Model file for the job. Use its own axes, mm. A direction names the side the tool comes from. Coordinates: 2 decimals unless noted, no trailing zeros. Loops run counter-clockwise (first coordinate to the right, second up) from the corner with the lowest first, then second, coordinate; pieces in that order, holes last. Notation, with made-up numbers: M -36,85 L 21,85 A25 ccw 21,109 Z; hole C 46.5,46 d8. An arc over 180 degrees is marked long. Write item = value, one per line. Start each with the question number.
Autodesk Inventor part; units mm, degrees
ref_plane "YZ Plane" through (0, 0, 0) normal (1, 0, 0) x (0, 1, 0)
ref_plane "XZ Plane" through (0, 0, 0) normal (0, 1, 0) x (-1, 0, 0)
ref_plane "XY Plane" through (0, 0, 0) normal (0, 0, 1) x (1, 0, 0)
sketch "Sketch1" plane through (0, 0, 0) normal (0, 0, 1) x (1, 0, 0)
  line L0 (-15.35, 11.85) -> (15.35, 11.85)
  line L1 (15.35, 11.85) -> (15.35, -11.85)
  line L2 (15.35, -11.85) -> (-15.35, -11.85)
  line L3 (-15.35, -11.85) -> (-15.35, 11.85)
  point P0 (0, 0)
  dimension "d0" = 30.7
  dimension "d2" = 23.7
  dimension "d3" = 15.35
  dimension "d4" = 11.85
extrude "Extrusion1" add sketch "Sketch1" against normal blind 3.2
sketch "Sketch2" plane through (0, 0, -3.2) normal (0, 0, -1) x (-1, 0, 0)
  line L0 (15.35, -11.85) -> (15.35, 11.85)
  line L1 (-11.25, 9.9) -> (11.25, 9.9)
  line L2 (13.25, 6.2453) -> (13.25, -5.9)
  line L3 (11.75, -9.9) -> (-11.75, -9.9)
  line L4 (-13.25, -5.9) -> (-13.25, 6.2453)
  line L5 (11.75, -9.9) -> (11.75, -9.0225)
  arc A0 (11.75, -9.0225) -> (13.25, -5.9) centre (9.25, -5.9) ccw
  line L6 (0, 0) -> (0, 2.1839)
  line L7 (-11.75, -9.9) -> (-11.75, -9.0225)
  arc A1 (-13.25, -5.9) -> (-11.75, -9.0225) centre (-9.25, -5.9) ccw
  line L8 (11.25, 9.9) -> (11.25, 7.4)
  line L9 (11.25, 7.4) -> (13.25, 6.2453)
  line L10 (-11.25, 9.9) -> (-11.25, 7.4)
  line L11 (-11.25, 7.4) -> (-13.25, 6.2453)
  dimension "d10" = 9.9
  dimension "d11" = 13.25
  dimension "d13" = 8
  dimension "d15" = 1.5
  dimension "d19" = 120
  dimension "d20" = 19.8
  dimension "d21" = 2
  dimension "d22" = 2.5
extrude "Extrusion2" add sketch "Sketch2" along normal blind 16
sketch "Sketch3" plane through (0, 0, -19.2) normal (0, 0, -1) x (-1, 0, 0)
  line L0 (-11.25, 9.9) -> (-11.25, 7.4)
  line L1 (-1.75, 7.5) -> (-1.75, -0.5)
  line L2 (-1.75, -0.5) -> (1.75, -0.5)
  line L3 (1.75, -0.5) -> (1.75, 7.5)
  line L4 (1.75, 7.5) -> (-1.75, 7.5)
  line L5 (-9.5, 2) -> (-9.5, -6)
  line L6 (-9.5, -6) -> (-6, -6)
  line L7 (-6, -6) -> (-6, 2)
  line L8 (-6, 2) -> (-9.5, 2)
  line L9 (6, 2) -> (6, -6)
  line L10 (6, -6) -> (9.5, -6)
  line L11 (9.5, -6) -> (9.5, 2)
  line L12 (9.5, 2) -> (6, 2)
  point P0 (0, 0)
  dimension "d25" = 3.5
  dimension "d27" = 8
  dimension "d28" = 1.75
  dimension "d29" = 7.5
  dimension "d30" = 3.5
  dimension "d31" = 8
  dimension "d32" = 3.5
  dimension "d33" = 8
  dimension "d34" = 2
  dimension "d35" = 2
  dimension "d36" = 6
  dimension "d37" = 6
extrude "Extrusion3" add sketch "Sketch3" along normal blind 1.5
sketch "Sketch4" plane through (0, 0, -20.7) normal (0, 0, -1) x (-1, 0, 0)
  line L0 (-6, -6) -> (-6, 2)
  line L1 (-6, 2) -> (-9.5, 2)
  line L2 (-8.25, 0) -> (-8.25, -4)
  line L3 (-8.25, -4) -> (-7.25, -4)
  line L4 (-7.25, -4) -> (-7.25, 0)
  line L5 (-7.25, 0) -> (-8.25, 0)
  point P0 (-9.5, -6)
  point P1 (0, 0)
  dimension "d40" = 4
  dimension "d42" = 1
  dimension "d43" = 1.25
  dimension "d44" = 3.5
  dimension "d45" = 8
  dimension "d46" = 2
extrude "Extrusion4" add sketch "Sketch4" along normal blind 5.5
sketch "Sketch6" plane through (0, 0, -20.7) normal (0, 0, -1) x (-1, 0, 0)
  line L0 (-1.75, -0.5) -> (1.75, -0.5)
  line L1 (1.75, -0.5) -> (1.75, 7.5)
  line L2 (1.75, 7.5) -> (-1.75, 7.5)
  line L3 (-0.5, 5.5) -> (0.5, 5.5)
  line L4 (0.5, 5.5) -> (0.5, 1.5)
  line L5 (0.5, 1.5) -> (-0.5, 1.5)
  line L6 (-0.5, 1.5) -> (-0.5, 5.5)
  point P0 (0, 0)
  dimension "d55" = 1
  dimension "d57" = 4
  dimension "d58" = 1.25
  dimension "d59" = 2
  dimension "d60" = 8
  dimension "d61" = 2
extrude "Extrusion5" add sketch "Sketch6" along normal blind 5.5
sketch "Sketch7" plane through (0, 0, -20.7) normal (0, 0, -1) x (-1, 0, 0)
  line L0 (9.5, -6) -> (9.5, 2)
  line L1 (9.5, 2) -> (6, 2)
  line L2 (8.25, -4) -> (7.25, -4)
  line L3 (7.25, -4) -> (7.25, 0)
  line L4 (7.25, 0) -> (8.25, 0)
  line L5 (8.25, 0) -> (8.25, -4)
  point P0 (0, 0)
  dimension "d64" = 2
  dimension "d65" = 4
  dimension "d66" = 1.25
  dimension "d67" = 1
extrude "Extrusion6" add sketch "Sketch7" along normal blind 5.5
sketch "Sketch8" plane through (8.25, -4, -20.7) normal (1, 0, 0) x (0, 0, -1)
  line L0 (0, 0) -> (0, 4)
  line L1 (0, 0) -> (5.5, 0)
  line L2 (5.5, 4) -> (5.5, 0)
  line L3 (0, 4) -> (5.5, 4)
  arc A0 (3.5, 0) -> (3.5, 4) centre (3.5, 2) ccw
  arc A1 (3.5, 0.9) -> (3.5, 3.1) centre (3.5, 2) ccw
  line L4 (3.5, 2) -> (2.8, 2)
  arc A2 (2.8, 3.1) -> (2.8, 0.9) centre (2.8, 2) ccw
  line L5 (2.8, 3.1) -> (3.5, 3.1)
  line L6 (3.5, 0.9) -> (2.8, 0.9)
  line L7 (3.5, 4) -> (5.5, 4)
  line L8 (5.5, 4) -> (5.5, 0)
  line L9 (5.5, 0) -> (3.5, 0)
  point P0 (-20.7, 4)
  dimension "d70" = 4
  dimension "d72" = 2.2
  dimension "d73" = 0.7
  dimension "d74" = 2.2
extrude "Extrusion7" cut sketch "Sketch8" against normal blind 1 contours A0 L2 L1 | L3 L2 A0 | L6 A2 L5 A1
sketch "Sketch11" plane through (0.5, 1.5, -20.7) normal (1, 0, 0) x (0, 0, -1)
  line L0 (0, 0) -> (0, 4)
  line L1 (0, 0) -> (5.5, 0)
  line L2 (5.5, 4) -> (5.5, 0)
  line L3 (0, 4) -> (5.5, 4)
  arc A0 (3.5, 0) -> (3.5, 4) centre (3.5, 2) ccw
  line L4 (3.5, 0) -> (5.5, 0)
  line L5 (5.5, 4) -> (5.5, 0)
  line L6 (5.5, 4) -> (3.5, 4)
  arc A1 (3.5, 0.9) -> (3.5, 3.1) centre (3.5, 2) ccw
  line L7 (3.5, 2) -> (2.8, 2)
  arc A2 (2.8, 3.1) -> (2.8, 0.9) centre (2.8, 2) ccw
  line L8 (2.8, 3.1) -> (3.5, 3.1)
  line L9 (3.5, 0.9) -> (2.8, 0.9)
  point P0 (-20.7, -1.5)
  dimension "d88" = 4
  dimension "d91" = 2.2
  dimension "d92" = 0.7
  dimension "d93" = 2.2
sketch "Sketch12" plane through (-7.25, -4, -20.7) normal (1, 0, 0) x (0, 0, -1)
  arc A0 (3.5, 0) -> (3.5, 4) centre (3.5, 2) ccw
  arc A1 (3.5, 0.9) -> (3.5, 3.1) centre (3.5, 2) ccw
  line L0 (3.5, 2) -> (2.8, 2)
  arc A2 (2.8, 3.1) -> (2.8, 0.9) centre (2.8, 2) ccw
  line L1 (2.8, 3.1) -> (3.5, 3.1)
  line L2 (3.5, 0.9) -> (2.8, 0.9)
  line L3 (0, 4) -> (5.5, 4)
  line L4 (5.5, 4) -> (5.5, 0)
  line L5 (5.5, 4) -> (3.5, 4)
  line L6 (3.5, 0) -> (5.5, 0)
  point P0 (-20.7, -1.5)
  dimension "d94" = 4
  dimension "d95" = 2.2
  dimension "d96" = 0.7
  dimension "d97" = 2.2
extrude "Extrusion8" cut sketch "Sketch11" against normal blind 1 contours A0 L2 L1 | L3 L2 A0 | L9 A2 L8 A1
extrude "Extrusion9" cut sketch "Sketch12" against normal blind 1 contours L2 A2 L1 A1
sketch "Sketch13" plane through (-7.25, -4, -20.7) normal (1, 0, 0) x (0, 0, -1)
  line L0 (0, 0) -> (5.5, 0)
  line L1 (5.5, 4) -> (5.5, 0)
  line L2 (0, 4) -> (5.5, 4)
  circle A0 centre (3.5, 2) radius 2
  line L3 (3.5, 4) -> (5.5, 4)
  line L4 (5.5, 0) -> (5.5, 4)
  line L5 (3.5, 0) -> (5.5, 0)
  point P0 (-20.7, 4)
  dimension "d102" = 4
extrude "Extrusion10" cut sketch "Sketch13" against normal blind 1 contours A0 L1 L0 | L2 L1 A0
sketch "Sketch14" plane through (0, 0, 0) normal (0, 0, 1) x (1, 0, 0)
  line L0 (12, -8) -> (-12, -8)
  line L1 (-7, 8) -> (7, 8)
  line L2 (12, 3) -> (12, -8)
  line L3 (7, 8) -> (12, 3)
  line L4 (0, 0) -> (0, 4.7583)
  line L5 (-7, 8) -> (-12, 3)
  line L6 (-12, -8) -> (-12, 3)
  dimension "d107" = 16
  dimension "d108" = 12
  dimension "d109" = 8
  dimension "d110" = 45
  dimension "d111" = 5
extrude "Extrusion11" cut sketch "Sketch14" against normal blind 16
fillet "Fillet1" radius 1.5 4 edges at (-15.35, 11.85, -1.6) (15.35, 11.85, -1.6) (15.35, -11.85, -1.6) (-15.35, -11.85, -1.6)
fillet "Fillet2" radius 2 2 edges at (-12, -8, -8) (12, -8, -8)
fillet "Fillet3" radius 1.5 4 edges at (-12, 3, -8) (-7, 8, -8) (7, 8, -8) (12, 3, -8)
fillet "Fillet4" radius 1 8 edges at (-14.9107, 11.4107, 0) (0, 11.85, 0) (14.9107, 11.4107, 0) (15.35, 0, 0) (14.9107, -11.4107, 0) (0, -11.85, 0) (-14.9107, -11.4107, 0) (-15.35, 0, 0)
properties part number "701W-X202"
Item 1: 3-axis set-ups, long thin cutter, end or side, ignore diameter. For faces 1 (the cylindrical face through (11.43, -7.4, -8.11)), 2 (the cylindrical face through (-7.7, -2, -25.3)), 3 (the flat face through (-13.25, 0, -11)), 4 (the flat face through (7.25, -2, -22)): which of +Z, -Z, +X, -X, +Y, -Y reach the whole face in a straight line?
Item 2: Pin check, flat tips, straight feed: pin 1 Ø2 at (y, z) = (9, -10.5) entering from -X; pin 2 Ø10 at (y, z) = (1.5, -13) entering from +X; pin 3 Ø1 at (y, z) = (4, -14) entering from -X. Stop position of each tip, or through.
Item 3: Cut at C-C (z = -17). Give the cut face in (x, y), plus the area to 3 significant figures.
Item 4: Pull direction Y, two halves, no side cores. Call faces 5 (the flat face through (9.5, -2, -20)), 6 (the cylindrical face through (-11.4, -7.43, -8.11)), 7 (the flat face through (12.24, 6.83, -11.09)): +Y half, -Y half, draft (parallel to the pull), parting line (faces both ways), or undercut.
Item 5: Probe L1, parallel to Y at x = -6, z = -10; L2, parallel to X at y = -7.25, z = -1.5; L3, parallel to X at y = -2.75, z = -21.25. List the from-to ranges inside material, lowest first.
Item 6: Cut at D-D (x = 9). Give the cut face in (y, z).
Item 7: Cut at A-A (z = -1.75). Give the cut face in (x, y).
Item 8: Cut at B-B (y = -4.5). Give the cut face in (x, z).
Reported:
q1.face_1 = +Z
q1.face_2 = +X, -X
q1.face_3 = -Z, -X, +Y, -Y
q1.face_4 = -Z, +Y, -Y
q2.pin_1 = -11.25
q2.pin_2 = 13.25
q2.pin_3 = -13.25
q3.outline = M -13.25,-5.9 A4 ccw -11.75,-9.02 L -11.75,-9.9 L 11.75,-9.9 L 11.75,-9.02 A4 ccw 13.25,-5.9 L 13.25,6.25 L 11.25,7.4 L 11.25,9.9 L -11.25,9.9 L -11.25,7.4 L -13.25,6.25 Z
q3.area = 507 mm^2
q4.face_5 = draft
q4.face_6 = undercut
q4.face_7 = +Y half
q5.L1 = -9.9 to -8, 8 to 9.9
q5.L2 = -15.35 to -11.56, 11.56 to 15.35
q5.L3 = -8.25 to -7.25, 7.25 to 8.25
q6.outline = M -11.85,-3.2 L -9.9,-3.2 L -9.9,-19.2 L -6,-19.2 L -6,-20.7 L 2,-20.7 L 2,-19.2 L 9.9,-19.2 L 9.9,-3.2 L 11.85,-3.2 L 11.85,-1 A1 ccw 10.85,0 L 6,0 L 6,-16 L -8,-16 L -8,0 L -10.85,0 A1 ccw -11.85,-1 Z
q7.outline = M -15.35,-10.35 A1.5 ccw -13.85,-11.85 L 13.85,-11.85 A1.5 ccw 15.35,-10.35 L 15.35,10.35 A1.5 ccw 13.85,11.85 L -13.85,11.85 A1.5 ccw -15.35,10.35 Z; hole M -12,-6 A2 ccw -10,-8 L 10,-8 A2 ccw 12,-6 L 12,2.38 A1.5 ccw 11.56,3.44 L 7.44,7.56 A1.5 ccw 6.38,8 L -6.38,8 A1.5 ccw -7.44,7.56 L -11.56,3.44 A1.5 ccw -12,2.38 Z
q8.outline = M -15.35,-3.2 L -13.25,-3.2 L -13.25,-19.2 L -9.5,-19.2 L -9.5,-20.7 L -6,-20.7 L -6,-19.2 L 6,-19.2 L 6,-20.7 L 9.5,-20.7 L 9.5,-19.2 L 13.25,-19.2 L 13.25,-3.2 L 15.35,-3.2 L 15.35,-1 A1 ccw 14.35,0 L 12,0 L 12,-16 L -12,-16 L -12,0 L -14.35,0 A1 ccw -15.35,-1 Z
